The model under review builds one solid part; all positions refer to its coordinate system, in mm. Face numbers are marked on the shaded views. A direction names the side the tool comes from. Round coordinates to 2 decimals unless told otherwise and drop trailing zeros. Write each loop counter-clockwise with the first axis right and the second up, starting at its lowest first coordinate (ties: lowest second). Pieces come first, ordered by that corner, then holes. Notation, with made-up numbers: (57.5, 27) -> (101.5, 27) arc R22 cw to (101.5, 65) -> close; hole circle Ø8 at (-19, -13.75). An arc over 180 degrees is marked (long way). Return JSON: item names as keys, results as strings. Group by question number.
1. Tool access review of the marked faces 1, 2 and 3: name each direction out of +Z, -Z, +X, -X, +Y, -Y from which nothing blocks a thin tool from reaching the whole face with its end or side.
2. Mouldability with a two-part tool opening along X and no side actions: class the marked faces 4, 5 and 6 as pulls with the +X half, pulls with the -X half, needs draft (parallel to the pull), parting line crosses it, or undercut.
3. Clearance check with flat-ended pins moving along their axes: P1, Ø5, axis at x = -24.5, y = 5, coming from the -Z side; P2, Ø3, axis at x = -7.5, z = 2, coming from the +Y side; P3, Ø1, axis at x = -3, z = -15, coming from the -Y side (3 decimals). State where each tip first meets the part, or that it passes through.
4. Take a section at B-B, the plane y = 13. Write out the cut boundary in (x, z), then the cut area to 3 significant figures.
5. For line 1 along Z through (x, y) = (20, 0); line 2 along Z through (x, y) = (-26.75, 0); line 3 along X through (y, z) = (14, -5.5), list the stretches that pass through material, from the lowest coordinate up. Write a range as from..to.
6. Take a section at D-D, the plane x = 8.5. Write out the cut boundary in (y, z).
7. Take a section at A-A, the plane x = -21.5. Write out the cut boundary in (y, z), then the cut area to 3 significant figures.
8. Take a section at C-C, the plane z = 14. Write out the cut boundary in (x, y).
Autodesk Inventor part; units mm, degrees
ref_plane "YZ Plane" through (0, 0, 0) normal (1, 0, 0) x (0, 1, 0)
ref_plane "XZ Plane" through (0, 0, 0) normal (0, 1, 0) x (-1, 0, 0)
ref_plane "XY Plane" through (0, 0, 0) normal (0, 0, 1) x (1, 0, 0)
sketch "Sketch1" plane through (0, 0, 0) normal (0, 0, 1) x (1, 0, 0)
  line L0 (0, 0) -> (5.5, 0)
  line L1 (5.5, 0) -> (5.5, 7)
  line L2 (5.5, 7) -> (0, 7)
  line L3 (0, 7) -> (0, 0)
  line L4 (5.5, 0) -> (25.5, 0)
  line L5 (25.5, 0) -> (25.5, 5)
  line L6 (25.5, 5) -> (5.5, 5)
  line L7 (5.5, 5) -> (5.5, 0)
  line L8 (0, 0) -> (-39.5, 0)
  line L9 (-39.5, 0) -> (-39.5, 20)
  line L10 (-39.5, 20) -> (0, 20)
  line L11 (0, 20) -> (0, 0)
  dimension "d0" = 5.5
  dimension "d1" = 7
  dimension "d2" = 5
  dimension "d3" = 20
  dimension "d5" = 39.5
  dimension "d6" = 20
revolve "Revolution1" add sketch "Sketch1" angle 360 about axis through (5.5, 0, 0) along (1, 0, 0)
sketch "Sketch2" plane through (25.5, 0, 0) normal (1, 0, 0) x (0, 0, -1)
  point P0 (0, 0)
  point P1 (0, 0)
hole "Hole1" at (25.5, 0, 0) direction (-1, 0, 0) diameter 3.242 depth 11.8 tip angle 118
sketch "Sketch3" plane through (-39.5, 0, 0) normal (-1, 0, 0) x (0, 0, 1)
  point P0 (0, 0)
  point P1 (0, 0)
hole "Hole2" at (-39.5, 0, 0) direction (1, 0, 0) diameter 6.647 depth 22.2 tip angle 118
sketch "Sketch4" plane through (0, 0, 0) normal (0, 1, 0) x (-1, 0, 0)
  line L0 (29.5, -20) -> (14.5, -20)
  line L1 (14.5, -20) -> (14.5, -18)
  line L2 (14.5, -18) -> (29.5, -18)
  line L3 (29.5, -18) -> (29.5, -20)
  line L4 (14.5, 20) -> (29.5, 20)
  line L5 (29.5, 20) -> (29.5, 18)
  line L6 (29.5, 18) -> (14.5, 18)
  line L7 (14.5, 18) -> (14.5, 20)
  line L8 (39.5, 20) -> (39.5, -20)
  point P0 (0, 0)
  dimension "d21" = 15
  dimension "d22" = 36
  dimension "d23" = 2
  dimension "d24" = 2
  dimension "d25" = 10
extrude "Extrusion1" cut sketch "Sketch4" along normal through all both and the other way through all
fillet "Fillet1" radius 0.5 1 edges at (0, -7, 0)
fillet "Fillet2" radius 0.4 1 edges at (5.5, -5, 0)
chamfer "Chamfer1" distance 0.5 angle 45 1 edges at (25.5, -5, 0)
chamfer "Chamfer2" distance 0.5 angle 45 1 edges at (5.5, -7, 0)
equation "\"d23\" = d24"
properties part number "Top_Lever Shaft" material "Stainless Steel"
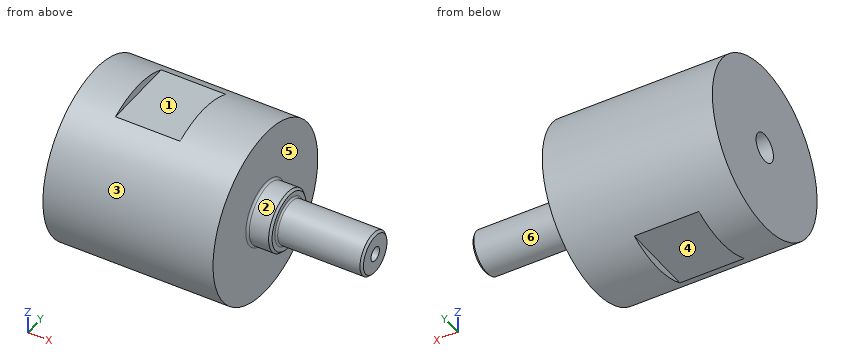
Output:
{
 "1": {"face 1": "+Z, +Y, -Y", "face 2": "+X", "face 3": "+X, -X"},
 "2": {"face 4": "undercut", "face 5": "pulls with the +X half", "face 6": "needs draft"},
 "3": {"P1": "stops at z = -18", "P2": "stops at y = 19.99", "P3": "stops at y = -13.775"},
 "4": {"outline": "(-39.5, -15.2) -> (0, -15.2) -> (0, 15.2) -> (-39.5, 15.2) -> close", "area": "1,200 mm^2"},
 "5": {"line 1": "z = -5..-1.62, 1.62..5", "line 2": "z = -18..-3.32, 3.32..18", "line 3": "x = -39.5..0"},
 "6": {"outline": "circle Ø10 at (0, 0)"},
 "7": {"outline": "(-8.72, -18) -> (8.72, -18) arc R20 ccw to (8.72, 18) -> (-8.72, 18) arc R20 ccw to start; hole circle Ø6.65 at (0, 0)", "area": "1,170 mm^2"},
 "8": {"outline": "(-39.5, -14.28) -> (0, -14.28) -> (0, 14.28) -> (-39.5, 14.28) -> close"}
}
